Source: CAD feature listing. Evaluate the final solid. Frame: model axes, mm. Round coordinates to 2 decimals unless told otherwise and drop trailing zeros. Write each loop counter-clockwise with the first axis right and the second up, starting at its lowest first coordinate (ties: lowest second). Pieces come first, ordered by that corner, then holes.
from build123d import *

# Parameters (mm, degrees)
SKETCH4_R           = 1.5
SKETCH4_R_2         = 19.05
SKETCH4_R_3         = 12.7
BOSS_EXTRUDE1_DEPTH = 3
SKETCH5_W           = 2.75
SKETCH5_H           = 6.096
LOWERSLOT_DEPTH     = 115.203880872
SKETCH5_3_W         = 2.75
SKETCH5_3_H         = 6.096
UPPERSLOT_DEPTH     = 115.203880872
LOWERSLOTS_COUNT    = 8
LOWERSLOTS_PITCH    = 12.7
UPPERSLOTS_COUNT    = 8
UPPERSLOTS_PITCH    = 12.7


with BuildPart() as part:
    # Sketch4 → Boss-Extrude1 (new, symmetric)
    # profile 1 of 4: a face of its own
    with BuildSketch(Plane(origin=(0, 0, 0), x_dir=(0, 0, -1), z_dir=(1, 0, 0))):
        with BuildLine():
            ThreePointArc((47.817596045, 22.032403955), (48.849976274, 23.577470153), (49.2125, 25.4))
            Line((49.2125, 25.4), (49.2125, 34.925))
            ThreePointArc((49.2125, 34.925), (47.817596045, 38.292596045), (44.45, 39.6875))
            Line((44.45, 39.6875), (-38.1, 39.6875))
            Line((-38.1, 39.6875), (-53.426606241, 25.4268804))
            Line((-53.426606241, 25.4268804), (-53.426606241, 1.775))
            ThreePointArc((-53.426606241, 1.775), (-56.426606241, -1.225), (-59.426606241, 1.775))
            Line((-59.426606241, 1.775), (-59.426606241, 19.84418869))
            Line((-59.426606241, 19.84418869), (-66.85, 12.937102224))
            Line((-66.85, 12.937102224), (-66.85, 8.3125))
            ThreePointArc((-66.85, 8.3125), (-69.423127317, 5.343025347), (-72.728519808, 7.467441591))
            Line((-72.728519808, 7.467441591), (-82.826645448, -1.928345458))
            ThreePointArc((-82.826645448, -1.928345458), (-62.244166574, 1.590789358), (-50.8, -15.875))
            ThreePointArc((-50.8, -15.875), (-61.330581006, -32.913837989), (-81.28, -31.115))
            Line((-81.28, -31.115), (-38.1, -63.5))
            Line((-38.1, -63.5), (43.992912904, -71.415514491))
            ThreePointArc((43.992912904, -71.415514491), (48.757334408, -68.706816071), (47.817596045, -63.307403955))
            Line((47.817596045, -63.307403955), (38.1, -53.589807909))
            Line((38.1, -53.589807909), (38.1, 12.314807909))
            Line((38.1, 12.314807909), (47.817596045, 22.032403955))
        make_face()
        with Locations((44.45, -66.675)):
            Circle(SKETCH4_R, mode=Mode.SUBTRACT)
        with Locations((44.45, 25.4)):
            Circle(SKETCH4_R, mode=Mode.SUBTRACT)
        with Locations((44.45, 34.925)):
            Circle(SKETCH4_R, mode=Mode.SUBTRACT)
    # profile 2 of 4: a face of its own
    with BuildSketch(Plane(origin=(0, 0, 0), x_dir=(0, 0, -1), z_dir=(1, 0, 0))):
        with Locations((-69.85, -15.875)):
            Circle(SKETCH4_R_2)
        with Locations((-69.85, -15.875)):
            Circle(SKETCH4_R_3, mode=Mode.SUBTRACT)
    # profile 3 of 4: a face of its own
    with BuildSketch(Plane(origin=(0, 0, 0), x_dir=(0, 0, -1), z_dir=(1, 0, 0))):
        with BuildLine():
            Line((-53.426606241, 1.775), (-53.426606241, 25.4268804))
            Line((-53.426606241, 25.4268804), (-59.426606241, 19.84418869))
            Line((-59.426606241, 19.84418869), (-59.426606241, 1.775))
            ThreePointArc((-59.426606241, 1.775), (-56.426606241, -1.225), (-53.426606241, 1.775))
        make_face()
    # profile 4 of 4: a face of its own
    with BuildSketch(Plane(origin=(0, 0, 0), x_dir=(0, 0, -1), z_dir=(1, 0, 0))):
        with BuildLine():
            Line((-66.85, 8.3125), (-66.85, 12.937102224))
            Line((-66.85, 12.937102224), (-72.728519808, 7.467441591))
            ThreePointArc((-72.728519808, 7.467441591), (-69.423127317, 5.343025347), (-66.85, 8.3125))
        make_face()
    extrude(amount=BOSS_EXTRUDE1_DEPTH, both=True)

    # Sketch5 → LowerSlot (cut, symmetric)
    with BuildSketch(Plane(origin=(3, 0, 0), x_dir=(0, 0, -1), z_dir=(1, 0, 0))):
        with Locations((34.29, -57.15)):
            Rectangle(SKETCH5_W, SKETCH5_H)
    lowerslot = extrude(amount=LOWERSLOT_DEPTH, both=True, mode=Mode.SUBTRACT)

    # Sketch5_3 → UpperSlot (cut, symmetric)
    with BuildSketch(Plane(origin=(3, 0, 0), x_dir=(0, 0, -1), z_dir=(1, 0, 0))):
        with Locations((-34.29, -57.15)):
            Rectangle(SKETCH5_3_W, SKETCH5_3_H)
    upperslot = extrude(amount=UPPERSLOT_DEPTH, both=True, mode=Mode.SUBTRACT)

    # LowerSlots: LowerSlot ×8
    with Locations(*[(0, i * LOWERSLOTS_PITCH, 0) for i in range(1, LOWERSLOTS_COUNT)]):
        add(lowerslot, mode=Mode.SUBTRACT)

    # UpperSlots: UpperSlot ×8
    with Locations(*[(0, i * UPPERSLOTS_PITCH, 0) for i in range(1, UPPERSLOTS_COUNT)]):
        add(upperslot, mode=Mode.SUBTRACT)


solid = part.part
1) Section query C-C on z = 31. Return the cut outline in (x, y), then the cut area to 3 significant figures.
Taken from the geometry:
outline: (-3, -64.18) - (3, -64.18) - (3, 39.69) - (-3, 39.69) - close
area: 623 mm2
2) Section query A-A on z = 69.85. Return the cut outline in (x, y) (1 decimal), then the cut area to 3 significant figures.
Taken from the geometry:
outline: (-3, -39.7) - (3, -39.7) - (3, -28.6) - (-3, -28.6) - close; (-3, -3.2) - (3, -3.2) - (3, 10.1) - (-3, 10.1) - close
area: 147 mm2
3) Material intervals for line 1 (Z direction, x = -0.3, y = 19.5) (3 decimals); line 2 (Z direction, x = 0.2, y = 6.5) (3 decimals); line 3 (Z direction, x = 1.65, y = -22) (3 decimals), sorted ascending.
Taken from the geometry:
line 1: z = -45.285 to -35.665, -32.915 to 32.915, 35.665 to 59.797
line 2: z = -38.1 to -35.665, -32.915 to 32.915, 35.665 to 73.768
line 3: z = -38.1 to -35.665, -32.915 to 32.915, 35.665 to 58.725, 80.975 to 87.888
4) Section query D-D on x = -1.7. State how many separate pieces and enclosed holes the cut face has, then the cut area to 3 significant figures.
Taken from the geometry:
separate pieces: 1
enclosed holes: 20
area: 10,800 mm2
5) Pull-direction query (Z, two-part tool) for faces 1 (the face through (3, -15, 21)), 2 (the face through (0, 19, 32.915)); classes: released by +Z, released by -Z, zero draft, split by the parting line, or undercut.
Taken from the geometry:
face 1: zero draft
face 2: undercut
6) Section query B-B on y = -57. Return the cut outline in (x, z) (3 decimals), then the cut area to 3 significant figures.
Taken from the geometry:
outline: (-3, -41.51) - (3, -41.51) - (3, -35.665) - (-3, -35.665) - close; (-3, -32.915) - (3, -32.915) - (3, 32.915) - (-3, 32.915) - close; (-3, 35.665) - (3, 35.665) - (3, 46.767) - (-3, 46.767) - close
area: 497 mm2
7) Contact query for flat-ended pins moving along their axis: P1, Ø1.8, axis at x = 1, y = 33.5, coming from the +Z side; P2, Ø1.8, axis at x = 1, y = -56, coming from the -Z side; P3, Ø3, axis at x = 0, y = -43.5, coming from the +Z side. Output: stop coordinate, or through.
Taken from the geometry:
P1: stops at z = 45.72
P2: stops at z = -41.41
P3: stops at z = 66.77
